Build history of the part. All positions in model axes, mm. Face numbers are marked on the shaded views. A direction names the side the tool comes from. Give positions to 0.01 mm unless a question says otherwise; leave off trailing zeros. Order: outer loops, then holes, each group sorted by start corner. A loop starts at its lowest first (then second) coordinate and runs counter-clockwise, first axis right, second up. Notation, with made-up numbers: (65.25, 77) - (116.25, 77) arc R16 ccw to (116.25, 95) - close; hole circle Ø3 at (77, -9). An arc over 180 degrees is marked (long way). Use a Markdown table: item, result. Add a question column.
(1) Slice it at D-D (z = -9.5). Write the cut outline in (x, y).
(2) Flat gauge pins, fed straight in: pin 1 (2.5 mm diameter, centred on x = 7, y = 17.5, fed in from -Z) (3 decimals); pin 2 (1 mm diameter, centred on x = 7.5, z = -10, fed in from +Y). Where does each tip first touch, or does it go through?
(3) Slice it at A-A (x = 5.85). Write the cut outline in (y, z) (3 decimals).
(4) Wall check: line 1 (Y direction, x = 6.75, z = -13); line 2 (Y direction, x = 2.75, z = -7.5); line 3 (Z direction, x = 6, y = 20.75) (3 decimals). Give the ranges that are in metal, low to high.
(5) Slice it at C-C (y = 15). Write the cut outline in (x, z) (3 decimals), then the cut area to 3 significant figures.
(6) Slice it at B-B (z = -7.25). Write the cut outline in (x, y).
(7) Which spindle directions (+Z, -Z, +X, -X, +Y, -Y) get a long thin tool onto all of the face, cutting with end or side? Do the marked faces 1, 2 and 3. Say none if no direction does.
from build123d import *

# Parameters (mm, degrees)
SKETCH1_W           = 11.7
SKETCH1_H           = 13.85
BOSS_EXTRUDE1_DEPTH = 6.2
SKETCH2_R           = 3.5
BOSS_EXTRUDE2_DEPTH = 7
BOSS_EXTRUDE3_DEPTH = 9


with BuildPart() as part:
    # Sketch1 → Boss-Extrude1 (new body)
    with BuildSketch(Plane(origin=(0, 0, 0), x_dir=(1, 0, 0), z_dir=(0, 1, 0))):
        with Locations((5.85, 6.925)):
            Rectangle(SKETCH1_W, SKETCH1_H)
    extrude(amount=BOSS_EXTRUDE1_DEPTH)

    # Sketch2 → Boss-Extrude2 (add)
    with BuildSketch(Plane(origin=(0, 6.2, 0), x_dir=(1, 0, 0), z_dir=(0, 1, 0))):
        with Locations((5.85, 6.925)):
            Circle(SKETCH2_R)
    extrude(amount=BOSS_EXTRUDE2_DEPTH)

    # Sketch3 → Boss-Extrude3 (add)
    with BuildSketch(Plane(origin=(0, 13.2, 0), x_dir=(1, 0, 0), z_dir=(0, 1, 0))):
        with BuildLine():
            Line((3.251923789, 8.425), (8.448076211, 8.425))
            ThreePointArc((8.448076211, 8.425), (5.85, 3.925), (3.251923789, 8.425))
        make_face()
    extrude(amount=BOSS_EXTRUDE3_DEPTH)


solid = part.part
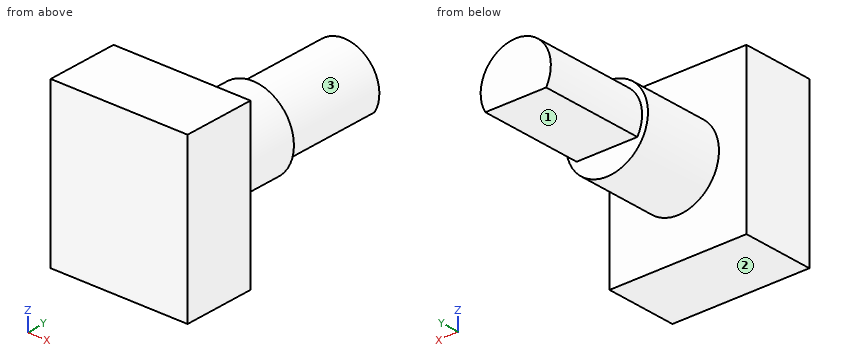
Solution:
| question | item | result |
|---|---|---|
| 1 | outline | (0, 0) - (11.7, 0) - (11.7, 6.2) - (8.22, 6.2) - (8.22, 13.2) - (3.48, 13.2) - (3.48, 6.2) - (0, 6.2) - close |
| 2 | pin 1 | z = -8.425 |
| 2 | pin 2 | y = 13.2 |
| 3 | outline | (0, -13.85) - (6.2, -13.85) - (6.2, -10.425) - (13.2, -10.425) - (13.2, -8.425) - (22.2, -8.425) - (22.2, -3.925) - (13.2, -3.925) - (13.2, -3.425) - (6.2, -3.425) - (6.2, 0) - (0, 0) - close |
| 4 | line 1 | 0 to 6.2 |
| 4 | line 2 | 0 to 13.2 |
| 4 | line 3 | -8.425 to -3.929 |
| 5 | outline | (3.252, -8.425) - (8.448, -8.425) arc R3 ccw (long way) to start |
| 5 | area | 22.7 mm2 |
| 6 | outline | (0, 0) - (11.7, 0) - (11.7, 6.2) - (9.33, 6.2) - (9.33, 13.2) - (8.83, 13.2) - (8.83, 22.2) - (2.87, 22.2) - (2.87, 13.2) - (2.37, 13.2) - (2.37, 6.2) - (0, 6.2) - close |
| 7 | face 1 | -Z, +X, -X, +Y |
| 7 | face 2 | -Z, +X, -X, +Y, -Y |
| 7 | face 3 | +Y |
